Autodesk Inventor part; units mm, degrees
ref_plane "YZ Plane" through (0, 0, 0) normal (1, 0, 0) x (0, 1, 0)
ref_plane "XZ Plane" through (0, 0, 0) normal (0, 1, 0) x (-1, 0, 0)
ref_plane "XY Plane" through (0, 0, 0) normal (0, 0, 1) x (1, 0, 0)
sketch "Sketch1" plane through (0, 0, 0) normal (0, 1, 0) x (-1, 0, 0)
  line L0 (0, 39) -> (7, 39)
  line L1 (7, 39) -> (7, 32)
  line L2 (7, 32) -> (0, 32)
  line L3 (0, 32) -> (0, 39)
  line L4 (7, -32) -> (0, -32)
  line L5 (0, -32) -> (0, -39)
  line L6 (0, -39) -> (7, -39)
  line L7 (7, -39) -> (7, -32)
  line L8 (7, 32) -> (7, -32) construction
  point P0 (0, 0)
  point P1 (7, 0)
  dimension "d0" = 78
  dimension "d1" = 7
extrude "Extrusion1" add sketch "Sketch1" along normal blind 2
sketch "Sketch2" plane through (0, 2, 0) normal (0, 1, 0) x (1, 0, 0)
  line L0 (-7, -32) -> (-7, -39)
  line L1 (0, 32) -> (0, 39)
  line L2 (-7, -34) -> (0, -34)
  line L3 (0, -34) -> (0, 34)
  line L4 (0, 34) -> (-7, 34)
  line L5 (-7, 34) -> (-7, -34)
  line L6 (0, -32) -> (-7, -32)
  line L7 (-7, 32) -> (0, 32)
  point P0 (0, 0)
  dimension "d4" = 2
  dimension "d5" = 2
extrude "Extrusion2" add sketch "Sketch2" along normal blind 4 contours L6 L3 L2 L0 | L5 L4 L1 L7
sketch "Sketch3" plane through (0, 6, 0) normal (0, 1, 0) x (1, 0, 0)
  line L0 (-7, -34) -> (0, -34)
  line L1 (0, 34) -> (-7, 34)
  line L2 (0, -34) -> (-7, -34)
  line L3 (-7, -34) -> (-7, 34)
  line L4 (-7, 34) -> (0, 34)
  line L5 (0, 34) -> (0, -34)
  point P0 (0, 0)
extrude "Extrusion3" add sketch "Sketch3" along normal blind 2
fillet "Fillet3" radius 1 9 edges at (-3.5, 2, 34) (-3.5, 2, 39) (-3.5, 2, -34) (-3.5, 0, 32) (-3.5, 0, -32) (-3.5, 6, -32) (-3.5, 6, 32) (-3.5, 8, -34) (-3.5, 8, 34)
fillet "Fillet4" radius 1 1 edges at (-3.5, 2, -39)
properties part number "neotrellis_support"
For this review, take the finished solid that the model builds, in its own axes (mm). A direction names the side the tool comes from. Coordinates: 2 decimals unless noted, no trailing zeros. Order: outer loops, then holes, each group sorted by start corner. A loop starts at its lowest first (then second) coordinate and runs counter-clockwise, first axis right, second up. Notation, with made-up numbers: (32.5, 50.5) - (62.5, 50.5) arc R22 ccw to (62.5, 86.5) - close; hole circle Ø1 at (18, 30.5). An arc over 180 degrees is marked (long way). Use one line per item in the form item = value.
Q1. For faces 4 (the flat face through (-4, 3, 32)), 5 (the flat face through (-3, 2, 37)), 6 (the flat face through (-3, 2, -36)), 7 (the flat face through (-7, 6.4, 0.2)), list the 3-axis set-ups (+Z, -Z, +X, -X, +Y, -Y) from which the entire face can be reached by the end or side of a thin tool; tool diameter is ignored.
Checked values:
face_4 = +X, -X, -Y
face_5 = +Z, +X, -X, +Y
face_6 = -Z, +X, -X, +Y
face_7 = +Z, -Z, -X, +Y, -Y
Q2. Draft analysis for pull direction Z (two halves, no side actions). For faces 1 (the flat face through (-4, 6, 0)), 2 (the flat face through (-4, 5, 34)), 3 (the flat face through (-4, 8, 0)), state which applies: +Z half, -Z half, draft (parallel to the pull), parting line (faces both ways), or undercut.
Checked values:
face_1 = undercut
face_2 = +Z half
face_3 = draft
Q3. Consider section C-C (z = 15). Give the boundary of the cut face in (x, y).
Checked values:
outline = (-7, 6) - (0, 6) - (0, 8) - (-7, 8) - close
Q4. For probe 1 along Z at (x, y) = (-2, 4.75); probe 2 along Z at (x, y) = (-3.25, 6.25); probe 3 along Z at (x, y) = (-3.75, 1), list the stretches that pass through material, from the lowest coordinate up. Write a range as from..to.
Checked values:
probe_1 = -34..-32, 32..34
probe_2 = -34..34
probe_3 = -39..-32, 32..39
Q5. Consider section B-B (x = -5). Give the boundary of the cut face in (y, z), then the cut area to 3 significant figures.
Checked values:
outline = (0, -39) - (1, -39) arc R1 ccw to (2, -38) - (2, -35) arc R1 cw to (3, -34) - (7, -34) arc R1 ccw to (8, -33) - (8, 33) arc R1 ccw to (7, 34) - (3, 34) arc R1 cw to (2, 35) - (2, 38) arc R1 ccw to (1, 39) - (0, 39) - (0, 33) arc R1 ccw to (1, 32) - (5, 32) arc R1 cw to (6, 31) - (6, -31) arc R1 cw to (5, -32) - (1, -32) arc R1 ccw to (0, -33) - close
area = 180 mm2
Q6. Consider section A-A (y = 4.25). Give the boundary of the cut face in (x, z), then the cut area to 3 significant figures.
Checked values:
outline = (-7, -34) - (0, -34) - (0, -32) - (-7, -32) - close; (-7, 32) - (0, 32) - (0, 34) - (-7, 34) - close
area = 28.0 mm2
Q7. For P1, Ø3, axis at x = -3, y = 4.5, coming from the -Z side; P2, Ø0.9, axis at x = -4, z = -36.5, coming from the +Y side; P3, Ø3, axis at x = -5, y = 3, coming from the +Z side, all flat-tipped, find the tip position at first contact; note any pin that passes through.
Checked values:
P1 = -34
P2 = 2
P3 = 38.87
